from build123d import *

# Parameters (mm, degrees)
CROQUIS1_W              = 38.1
CROQUIS1_H              = 6.31
SALIENTE_EXTRUIR1_DEPTH = 238.06
CROQUIS2_W              = 38.1
CROQUIS2_H              = 6.31
SALIENTE_EXTRUIR2_DEPTH = 489.1
CROQUIS3_W              = 38.1
CROQUIS3_H              = 6.31
SALIENTE_EXTRUIR3_DEPTH = 552.5
CROQUIS4_W              = 38.1
CROQUIS4_H              = 6.31
SALIENTE_EXTRUIR4_DEPTH = 324.39
CROQUIS5_R              = 6.35
CORTAR_EXTRUIR1_DEPTH   = 6.31


with BuildPart() as part:
    # Croquis1 → Saliente-Extruir1 (new body)
    with BuildSketch(Plane.XY):
        Rectangle(CROQUIS1_W, CROQUIS1_H)
    extrude(amount=SALIENTE_EXTRUIR1_DEPTH)

    # Croquis2 → Saliente-Extruir2 (add)
    with BuildSketch(Plane.XZ.offset(3.155)):
        with Locations((0, 234.905)):
            Rectangle(CROQUIS2_W, CROQUIS2_H)
    extrude(amount=SALIENTE_EXTRUIR2_DEPTH)

    # Croquis3 → Saliente-Extruir3 (add)
    with BuildSketch(Plane.XY.offset(238.06)):
        with Locations((0, -489.1)):
            Rectangle(CROQUIS3_W, CROQUIS3_H)
    extrude(amount=SALIENTE_EXTRUIR3_DEPTH)

    # Croquis4 → Saliente-Extruir4 (add)
    with BuildSketch(Plane(origin=(0, -485.945, 0), x_dir=(1, 0, 0), z_dir=(0, 1, 0))):
        with Locations((0, -787.405)):
            Rectangle(CROQUIS4_W, CROQUIS4_H)
    extrude(amount=SALIENTE_EXTRUIR4_DEPTH)

    # Croquis5 → Cortar-Extruir1 (cut)
    with BuildSketch(Plane.XY.offset(790.56)):
        with Locations((0, -173.447204666)):
            Circle(CROQUIS5_R)
        with Locations((0, -205.447204666)):
            Circle(CROQUIS5_R)
    extrude(amount=-CORTAR_EXTRUIR1_DEPTH, mode=Mode.SUBTRACT)


solid = part.part
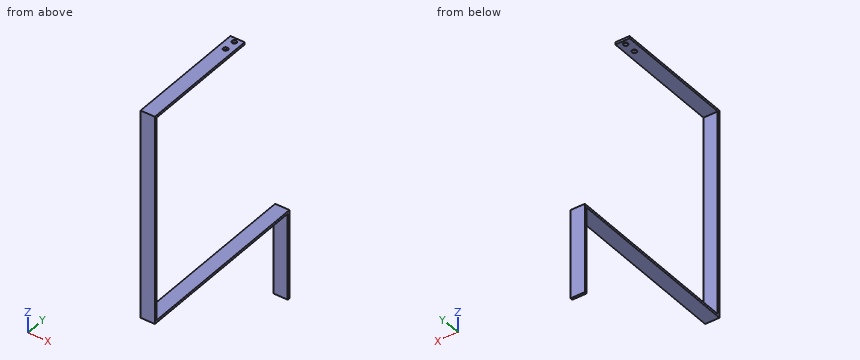
Geometry check sheet. Reference: the model listing, model coordinates, mm. Round coordinates to 2 decimals unless told otherwise and drop trailing zeros. Order: outer loops, then holes, each group sorted by start corner. A loop starts at its lowest first (then second) coordinate and runs counter-clockwise, first axis right, second up. Notation, with made-up numbers: (-31, 75.5) - (-22, 75.5) arc R29 cw to (-22, 99.5) - close; hole circle Ø8 at (66.25, 7). An arc over 180 degrees is marked (long way). One line per question, with ' | ' between items. Start each with the question number.
(1) Depth check by flat-ended pin: pin 1 Ø11.5 at (x, z) = (7, 603) entering from +Y (3 decimals); pin 2 Ø16.5 at (x, y) = (0, -205.45) entering from -Z; pin 3 Ø14.5 at (x, y) = (0, -173.45) entering from +Z; pin 4 Ø1.9 at (x, z) = (-7.5, 786.5) entering from +Y (3 decimals). Enter the tip coordinate at first touch or a pass-through.
(2) Sectioned sample at C-C on z = 201.5. Record the cut outline in (x, y) (3 decimals).
(3) Thickness scan on L1, parallel to Y at x = 0, z = 789.5 (3 decimals); L2, parallel to Z at x = -16, y = -318.5; L3, parallel to Z at x = 8.5, y = -112. Record the ranges inside material, lowest first. Write a range as [from, to].
(4) Sectioned sample at B-B on y = -245.5. Record the cut outline in (x, z), and give its area (3 significant figures).
(5) Sectioned sample at A-A on x = 0. Record the cut outline in (y, z) (3 decimals).
Conclusion:
1) pin 1: stops at y = -485.945 | pin 2: stops at z = 231.75 | pin 3: stops at z = 790.56 | pin 4: stops at y = -161.555
2) outline: (-19.05, -3.155) - (19.05, -3.155) - (19.05, 3.155) - (-19.05, 3.155) - close
3) L1: y = [-492.255, -211.797], [-199.097, -179.797], [-167.097, -161.555] | L2: z = [231.75, 238.06], [784.25, 790.56] | L3: z = [231.75, 238.06]
4) outline: (-19.05, 231.75) - (19.05, 231.75) - (19.05, 238.06) - (-19.05, 238.06) - close; (-19.05, 784.25) - (19.05, 784.25) - (19.05, 790.56) - (-19.05, 790.56) - close | area: 481 mm2
5) outline: (-492.255, 231.75) - (-3.155, 231.75) - (-3.155, 0) - (3.155, 0) - (3.155, 238.06) - (-485.945, 238.06) - (-485.945, 784.25) - (-211.797, 784.25) - (-211.797, 790.56) - (-492.255, 790.56) - close; (-199.097, 784.25) - (-179.797, 784.25) - (-179.797, 790.56) - (-199.097, 790.56) - close; (-167.097, 784.25) - (-161.555, 784.25) - (-161.555, 790.56) - (-167.097, 790.56) - close
